from build123d import *

# Parameters (mm, degrees)
SKETCH1_W           = 13
SKETCH1_H           = 10
BOSS_EXTRUDE1_DEPTH = 3
SKETCH2_W           = 3
SKETCH2_H           = 2
SKETCH2_H_2         = 3
CUT_EXTRUDE1_DEPTH  = 3
SKETCH3_W           = 3
SKETCH3_H           = 2
SKETCH3_H_2         = 3
CUT_EXTRUDE2_DEPTH  = 3


with BuildPart() as part:
    # Sketch1 → Boss-Extrude1 (new body)
    with BuildSketch(Plane.XY):
        Rectangle(SKETCH1_W, SKETCH1_H)
    extrude(amount=BOSS_EXTRUDE1_DEPTH)

    # Sketch2 → Cut-Extrude1 (cut)
    with BuildSketch(Plane.XY.offset(3)):
        with Locations((-5, 4)):
            Rectangle(SKETCH2_W, SKETCH2_H)
        with Locations((-5, 0)):
            Rectangle(SKETCH2_W, SKETCH2_H_2)
        with Locations((-5, -4)):
            Rectangle(SKETCH2_W, SKETCH2_H)
    extrude(amount=-CUT_EXTRUDE1_DEPTH, mode=Mode.SUBTRACT)

    # Sketch3 → Cut-Extrude2 (cut)
    with BuildSketch(Plane.XY.offset(3)):
        with Locations((5, 4)):
            Rectangle(SKETCH3_W, SKETCH3_H)
        with Locations((5, 0)):
            Rectangle(SKETCH3_W, SKETCH3_H_2)
        with Locations((5, -4)):
            Rectangle(SKETCH3_W, SKETCH3_H)
    extrude(amount=-CUT_EXTRUDE2_DEPTH, mode=Mode.SUBTRACT)


solid = part.part
Check sheet for the modelled part. Datum: model origin and axes. Units: mm. A direction names the side the tool comes from. Give positions to 0.01 mm unless a question says otherwise; leave off trailing zeros. Loops run counter-clockwise (first coordinate to the right, second up) from the corner with the lowest first, then second, coordinate; pieces in that order, holes last. Notation, with made-up numbers: M 88.5,-25 L 141.5,-25 A23 cw 141.5,-9 Z; hole C 79.25,65.25 d6. An arc over 180 degrees is marked long. Answer as a JSON object with one key per item and string values. Group by question number.
Q1. Material ranges on line 1 along Y through (x, z) = (5.5, 2.05); line 2 along X through (y, z) = (-4.5, 1.3), recorded low to high. Write a range as [from, to].
Q2. Cross-section at A-A on x = 5.75. Record the cut outline in (y, z), then the cut area to 3 significant figures.
Q3. Release check for a two-part mould opening along Y. For faces 1 (the flat face through (-3.5, 0, 2)), 2 (the flat face through (-5, -3, 2)), 3 (the flat face through (0, 0, 0)) record: released by +Y, released by -Y, zero draft, split by the parting line, or undercut.
Q4. Access from +Z, -Z, +X, -X, +Y, -Y to the whole of each face (thin tool, end or side, straight path). Record for faces 4 (the flat face through (5, -3, 2)), 5 (the flat face through (3.5, 0, 2)), 6 (the flat face through (3.5, 4, 2)), 7 (the flat face through (-3.5, 4, 2)).
Q5. Go/stop test with flat-tipped pins: P1, Ø1.5, axis at x = -5, z = 1, coming from the +Y side; P2, Ø1.5, axis at x = -4.5, z = 2, coming from the -Y side; P3, Ø0.6, axis at y = 4, z = 2, coming from the +X side. Record where each tip stops, or that it passes through.
Q6. Cross-section at B-B on z = 2.35. Record the cut outline in (x, y), then the cut area to 3 significant figures.
Q7. Cross-section at C-C on y = 3.5. Record the cut outline in (x, z), then the cut area to 3 significant figures.
Evaluation:
{
 "1": {"line 1": "y = [-3, -1.5], [1.5, 3]", "line 2": "x = [-3.5, 3.5]"},
 "2": {"outline": "M -3,0 L -1.5,0 L -1.5,3 L -3,3 Z; M 1.5,0 L 3,0 L 3,3 L 1.5,3 Z", "area": "9.00 mm2"},
 "3": {"face 1": "undercut", "face 2": "released by -Y", "face 3": "zero draft"},
 "4": {"face 4": "+Z, -Z, +X, -Y", "face 5": "+Z, -Z, +X", "face 6": "+Z, -Z, +X, +Y", "face 7": "+Z, -Z, -X, +Y"},
 "5": {"P1": "stops at y = 3", "P2": "stops at y = -3", "P3": "stops at x = 3.5"},
 "6": {"outline": "M -6.5,-3 L -3.5,-3 L -3.5,-5 L 3.5,-5 L 3.5,-3 L 6.5,-3 L 6.5,-1.5 L 3.5,-1.5 L 3.5,1.5 L 6.5,1.5 L 6.5,3 L 3.5,3 L 3.5,5 L -3.5,5 L -3.5,3 L -6.5,3 L -6.5,1.5 L -3.5,1.5 L -3.5,-1.5 L -6.5,-1.5 Z", "area": "88.0 mm2"},
 "7": {"outline": "M -3.5,0 L 3.5,0 L 3.5,3 L -3.5,3 Z", "area": "21.0 mm2"}
}
